from build123d import *

# Parameters (mm, degrees)
SKETCH1_W                 = 127.8
SKETCH1_H                 = 85.5
BOSS_EXTRUDE1_DEPTH       = 2.1
SKETCH2_R                 = 1.9
CUT_EXTRUDE1_DEPTH        = 154.777436576
LPATTERN1_COUNT           = 3
LPATTERN1_PITCH           = 59.9
MIRROR1_COPY_1_SKETCH_R   = 1.9
MIRROR1_COPY_1_DEPTH      = 154.777436576
MIRROR1_COPY_2_SKETCH_R   = 1.9
MIRROR1_COPY_2_DEPTH      = 154.777436576
SKETCH3_W                 = 3
SKETCH3_H                 = 1.5
BOSS_EXTRUDE2_DEPTH       = 1.9
LPATTERN2_COUNT           = 4
LPATTERN2_PITCH           = 9
MIRROR2_COPY_1_SKETCH_W   = 3
MIRROR2_COPY_1_SKETCH_H   = 1.5
MIRROR2_COPY_1_DEPTH      = 1.9
MIRROR2_COPY_2_SKETCH_W   = 3
MIRROR2_COPY_2_SKETCH_H   = 1.5
MIRROR2_COPY_2_DEPTH      = 1.9
MIRROR2_COPY_3_SKETCH_W   = 3
MIRROR2_COPY_3_SKETCH_H   = 1.5
MIRROR2_COPY_3_DEPTH      = 1.9
LPATTERN3_COUNT           = 2
LPATTERN3_PITCH           = 54
LPATTERN3_COPY_1_SKETCH_W = 3
LPATTERN3_COPY_1_SKETCH_H = 1.5
LPATTERN3_COPY_1_DEPTH    = 1.9
LPATTERN3_COPY_2_SKETCH_W = 3
LPATTERN3_COPY_2_SKETCH_H = 1.5
LPATTERN3_COPY_2_DEPTH    = 1.9
LPATTERN3_COPY_3_SKETCH_W = 3
LPATTERN3_COPY_3_SKETCH_H = 1.5
LPATTERN3_COPY_3_DEPTH    = 1.9
LPATTERN3_COPY_4_SKETCH_W = 3
LPATTERN3_COPY_4_SKETCH_H = 1.5
LPATTERN3_COPY_4_DEPTH    = 1.9
LPATTERN3_COPY_5_SKETCH_W = 3
LPATTERN3_COPY_5_SKETCH_H = 1.5
LPATTERN3_COPY_5_DEPTH    = 1.9
LPATTERN3_COPY_6_SKETCH_W = 3
LPATTERN3_COPY_6_SKETCH_H = 1.5
LPATTERN3_COPY_6_DEPTH    = 1.9
LPATTERN3_COPY_7_SKETCH_W = 3
LPATTERN3_COPY_7_SKETCH_H = 1.5
LPATTERN3_COPY_7_DEPTH    = 1.9
SKETCH4_W                 = 1.5
SKETCH4_H                 = 3
BOSS_EXTRUDE3_DEPTH       = 1.9
LPATTERN4_COUNT           = 8
LPATTERN4_PITCH           = 9


with BuildPart() as part:
    # Sketch1 → Boss-Extrude1 (new body)
    with BuildSketch(Plane(origin=(0, 0, 0), x_dir=(1, 0, 0), z_dir=(0, 1, 0))):
        with Locations((63.9, 42.75)):
            Rectangle(SKETCH1_W, SKETCH1_H)
    extrude(amount=BOSS_EXTRUDE1_DEPTH)

    # Sketch2 → Cut-Extrude1 (cut, through all)
    with BuildSketch(Plane(origin=(0, 2.1, 0), x_dir=(1, 0, 0), z_dir=(0, 1, 0))):
        with Locations(Location((4, 3, 0), (0, 0, 270))):
            Circle(SKETCH2_R)
    cut_extrude1 = extrude(amount=-CUT_EXTRUDE1_DEPTH, mode=Mode.SUBTRACT)

    # LPattern1: Cut-Extrude1 ×3
    with Locations(*[(i * LPATTERN1_PITCH, 0, 0) for i in range(1, LPATTERN1_COUNT)]):
        add(cut_extrude1, mode=Mode.SUBTRACT)

    # Mirror1: Cut-Extrude1 across plane
    add(cut_extrude1.mirror(Plane.XY.offset(-42.75)), mode=Mode.SUBTRACT)

    # Mirror1 copy 1 sketch → Mirror1 copy 1 (cut, through all)
    with BuildSketch(Plane(origin=(59.9, 2.1, -85.5), x_dir=(1, 0, 0), z_dir=(0, 1, 0))):
        with Locations((4, -3)):
            Circle(MIRROR1_COPY_1_SKETCH_R)
    extrude(amount=-MIRROR1_COPY_1_DEPTH, mode=Mode.SUBTRACT)

    # Mirror1 copy 2 sketch → Mirror1 copy 2 (cut, through all)
    with BuildSketch(Plane(origin=(119.8, 2.1, -85.5), x_dir=(1, 0, 0), z_dir=(0, 1, 0))):
        with Locations((4, -3)):
            Circle(MIRROR1_COPY_2_SKETCH_R)
    extrude(amount=-MIRROR1_COPY_2_DEPTH, mode=Mode.SUBTRACT)

    # Sketch3 → Boss-Extrude2 (add)
    with BuildSketch(Plane(origin=(0, 2.1, 0), x_dir=(1, 0, 0), z_dir=(0, 1, 0))):
        with Locations((77.5, 41.25)):
            Rectangle(SKETCH3_W, SKETCH3_H)
        with Locations((77.5, 35.25)):
            Rectangle(SKETCH3_W, SKETCH3_H)
    boss_extrude2 = extrude(amount=BOSS_EXTRUDE2_DEPTH)

    # LPattern2: Boss-Extrude2 ×4
    with Locations(*[(0, 0, i * LPATTERN2_PITCH) for i in range(1, LPATTERN2_COUNT)]):
        add(boss_extrude2)

    # Mirror2: Boss-Extrude2 across plane
    add(boss_extrude2.mirror(Plane.XY.offset(-42.75)))

    # Mirror2 copy 1 sketch → Mirror2 copy 1 (add)
    with BuildSketch(Plane(origin=(0, 2.1, -94.5), x_dir=(1, 0, 0), z_dir=(0, 1, 0))):
        with Locations((77.5, -41.25)):
            Rectangle(MIRROR2_COPY_1_SKETCH_W, MIRROR2_COPY_1_SKETCH_H)
        with Locations((77.5, -35.25)):
            Rectangle(MIRROR2_COPY_1_SKETCH_W, MIRROR2_COPY_1_SKETCH_H)
    extrude(amount=MIRROR2_COPY_1_DEPTH)

    # Mirror2 copy 2 sketch → Mirror2 copy 2 (add)
    with BuildSketch(Plane(origin=(0, 2.1, -103.5), x_dir=(1, 0, 0), z_dir=(0, 1, 0))):
        with Locations((77.5, -41.25)):
            Rectangle(MIRROR2_COPY_2_SKETCH_W, MIRROR2_COPY_2_SKETCH_H)
        with Locations((77.5, -35.25)):
            Rectangle(MIRROR2_COPY_2_SKETCH_W, MIRROR2_COPY_2_SKETCH_H)
    extrude(amount=MIRROR2_COPY_2_DEPTH)

    # Mirror2 copy 3 sketch → Mirror2 copy 3 (add)
    with BuildSketch(Plane(origin=(0, 2.1, -112.5), x_dir=(1, 0, 0), z_dir=(0, 1, 0))):
        with Locations((77.5, -41.25)):
            Rectangle(MIRROR2_COPY_3_SKETCH_W, MIRROR2_COPY_3_SKETCH_H)
        with Locations((77.5, -35.25)):
            Rectangle(MIRROR2_COPY_3_SKETCH_W, MIRROR2_COPY_3_SKETCH_H)
    extrude(amount=MIRROR2_COPY_3_DEPTH)

    # LPattern3: Boss-Extrude2 ×2
    with Locations(*[(-i * LPATTERN3_PITCH, 0, 0) for i in range(1, LPATTERN3_COUNT)]):
        add(boss_extrude2)

    # LPattern3 copy 1 sketch → LPattern3 copy 1 (add)
    with BuildSketch(Plane(origin=(-54, 2.1, 9), x_dir=(1, 0, 0), z_dir=(0, 1, 0))):
        with Locations((77.5, 41.25)):
            Rectangle(LPATTERN3_COPY_1_SKETCH_W, LPATTERN3_COPY_1_SKETCH_H)
        with Locations((77.5, 35.25)):
            Rectangle(LPATTERN3_COPY_1_SKETCH_W, LPATTERN3_COPY_1_SKETCH_H)
    extrude(amount=LPATTERN3_COPY_1_DEPTH)

    # LPattern3 copy 2 sketch → LPattern3 copy 2 (add)
    with BuildSketch(Plane(origin=(-54, 2.1, 18), x_dir=(1, 0, 0), z_dir=(0, 1, 0))):
        with Locations((77.5, 41.25)):
            Rectangle(LPATTERN3_COPY_2_SKETCH_W, LPATTERN3_COPY_2_SKETCH_H)
        with Locations((77.5, 35.25)):
            Rectangle(LPATTERN3_COPY_2_SKETCH_W, LPATTERN3_COPY_2_SKETCH_H)
    extrude(amount=LPATTERN3_COPY_2_DEPTH)

    # LPattern3 copy 3 sketch → LPattern3 copy 3 (add)
    with BuildSketch(Plane(origin=(-54, 2.1, 27), x_dir=(1, 0, 0), z_dir=(0, 1, 0))):
        with Locations((77.5, 41.25)):
            Rectangle(LPATTERN3_COPY_3_SKETCH_W, LPATTERN3_COPY_3_SKETCH_H)
        with Locations((77.5, 35.25)):
            Rectangle(LPATTERN3_COPY_3_SKETCH_W, LPATTERN3_COPY_3_SKETCH_H)
    extrude(amount=LPATTERN3_COPY_3_DEPTH)

    # LPattern3 copy 4 sketch → LPattern3 copy 4 (add)
    with BuildSketch(Plane(origin=(-54, 2.1, -85.5), x_dir=(1, 0, 0), z_dir=(0, 1, 0))):
        with Locations((77.5, -41.25)):
            Rectangle(LPATTERN3_COPY_4_SKETCH_W, LPATTERN3_COPY_4_SKETCH_H)
        with Locations((77.5, -35.25)):
            Rectangle(LPATTERN3_COPY_4_SKETCH_W, LPATTERN3_COPY_4_SKETCH_H)
    extrude(amount=LPATTERN3_COPY_4_DEPTH)

    # LPattern3 copy 5 sketch → LPattern3 copy 5 (add)
    with BuildSketch(Plane(origin=(-54, 2.1, -94.5), x_dir=(1, 0, 0), z_dir=(0, 1, 0))):
        with Locations((77.5, -41.25)):
            Rectangle(LPATTERN3_COPY_5_SKETCH_W, LPATTERN3_COPY_5_SKETCH_H)
        with Locations((77.5, -35.25)):
            Rectangle(LPATTERN3_COPY_5_SKETCH_W, LPATTERN3_COPY_5_SKETCH_H)
    extrude(amount=LPATTERN3_COPY_5_DEPTH)

    # LPattern3 copy 6 sketch → LPattern3 copy 6 (add)
    with BuildSketch(Plane(origin=(-54, 2.1, -103.5), x_dir=(1, 0, 0), z_dir=(0, 1, 0))):
        with Locations((77.5, -41.25)):
            Rectangle(LPATTERN3_COPY_6_SKETCH_W, LPATTERN3_COPY_6_SKETCH_H)
        with Locations((77.5, -35.25)):
            Rectangle(LPATTERN3_COPY_6_SKETCH_W, LPATTERN3_COPY_6_SKETCH_H)
    extrude(amount=LPATTERN3_COPY_6_DEPTH)

    # LPattern3 copy 7 sketch → LPattern3 copy 7 (add)
    with BuildSketch(Plane(origin=(-54, 2.1, -112.5), x_dir=(1, 0, 0), z_dir=(0, 1, 0))):
        with Locations((77.5, -41.25)):
            Rectangle(LPATTERN3_COPY_7_SKETCH_W, LPATTERN3_COPY_7_SKETCH_H)
        with Locations((77.5, -35.25)):
            Rectangle(LPATTERN3_COPY_7_SKETCH_W, LPATTERN3_COPY_7_SKETCH_H)
    extrude(amount=LPATTERN3_COPY_7_DEPTH)

    # Sketch4 → Boss-Extrude3 (add)
    with BuildSketch(Plane(origin=(0, 2.1, 0), x_dir=(1, 0, 0), z_dir=(0, 1, 0))):
        with Locations((18.25, 74.25)):
            Rectangle(SKETCH4_W, SKETCH4_H)
    boss_extrude3 = extrude(amount=BOSS_EXTRUDE3_DEPTH)

    # LPattern4: Boss-Extrude3 ×8
    with Locations(*[(0, 0, i * LPATTERN4_PITCH) for i in range(1, LPATTERN4_COUNT)]):
        add(boss_extrude3)


solid = part.part
Check sheet for the modelled part. Datum: model origin and axes. Units: mm. Round coordinates to 2 decimals unless told otherwise and drop trailing zeros. Loops run counter-clockwise (first coordinate to the right, second up) from the corner with the lowest first, then second, coordinate; pieces in that order, holes last. Notation, with made-up numbers: M 50,23 L 72,23 A3 cw 72,27 Z; hole C 74,20.5 d7. An arc over 180 degrees is marked long. One line per question, with ' | ' between items. Start each with the question number.
Item 1: Gauge pin test, flat ends, axial feed: pin 1 Ø0.8 at (x, y) = (18, 3) entering from -Z; pin 2 Ø1.2 at (y, z) = (3, -77.5) entering from +X; pin 3 Ø1.5 at (x, y) = (24, 3.5) entering from -Z. Record the tip position at first contact, or that the pin passes through.
Item 2: Release check for a two-part mould opening along Z. For faces 1 (the face through (123.072, 1.065, -1.245)), 2 (the face through (63, 0, -43)), 3 (the face through (5.602, 1.065, -1.979)) record: released by +Z, released by -Z, zero draft, split by the parting line, or undercut.
Item 3: Section check A-A (x = 4). Record the boundary of the cut face in (y, z).
Item 4: Section check B-B (z = -3). Record the boundary of the cut face in (x, y), and give its area (3 significant figures).
Item 5: Section check C-C (x = 83.5). Record the boundary of the cut face in (y, z), and give its area (3 significant figures).
Item 6: Scan lines: probe 1 along X at (y, z) = (0.55, -82.5); probe 2 along X at (y, z) = (2.65, -68.5); probe 3 along Y at (x, z) = (115, -70). Record each from-to range of solid material in increasing order.
Worked out:
1) pin 1: z = -75.75 | pin 2: x = 79 | pin 3: z = -78
2) face 1: undercut | face 2: zero draft | face 3: undercut
3) outline: M 0,-85.5 L 2.1,-85.5 L 2.1,-84.4 L 0,-84.4 Z; M 0,-80.6 L 2.1,-80.6 L 2.1,-4.9 L 0,-4.9 Z; M 0,-1.1 L 2.1,-1.1 L 2.1,0 L 0,0 Z
4) outline: M 0,0 L 2.1,0 L 2.1,2.1 L 0,2.1 Z; M 5.9,0 L 62,0 L 62,2.1 L 5.9,2.1 Z; M 65.8,0 L 121.9,0 L 121.9,2.1 L 65.8,2.1 Z; M 125.7,0 L 127.8,0 L 127.8,2.1 L 125.7,2.1 Z | area: 244 mm^2
5) outline: M 0,-85.5 L 2.1,-85.5 L 2.1,0 L 0,0 Z | area: 180 mm^2
6) probe 1: 0 to 2.1, 5.9 to 62, 65.8 to 121.9, 125.7 to 127.8 | probe 2: 22 to 25, 76 to 79 | probe 3: 0 to 2.1
